For this review, use the dimensioned drawing (mm, ordinates from the lowest corner) and the shaded views. A direction names the side the tool comes from. Round coordinates to 2 decimals unless told otherwise and drop trailing zeros. Write each loop counter-clockwise with the first axis right and the second up, starting at its lowest first coordinate (ties: lowest second). Pieces come first, ordered by that corner, then holes. Notation, with made-up numbers: M 9,53 L 28,53 A22 cw 28,60 Z; hole C 10,9 d9. An arc over 180 degrees is marked long. One line per question, with ' | ' between items. Start each with the question number.
Item 1: For L1, parallel to X at y = 12.25, z = 15.5; L2, parallel to X at y = 0.55, z = 32, list the stretches that pass through material, from the lowest coordinate up.
Item 2: Machinability: for the marked faces 1 and 2, which of the approach directions +Z, -Z, +X, -X, +Y, -Y give a long, thin tool a straight path to every point of the face, cutting with its end or side? Answer none if there is none.
Item 3: Add section C-C, the plane y = 9.75. State the section outline as (x, z) points.
Item 4: Insertion check: pin 1 Ø5 at (y, z) = (16, 31.5) entering from -X; pin 2 Ø5.5 at (x, z) = (7, 57) entering from +Y. Each pin has a flat end and moves straight along its axis. Give the tip position at first contact, or say it passes through.
Item 5: Add section B-B, the plane x = 32. State the section outline as (y, z) points.
Item 6: Add section A-A, the plane z = 32. State the section outline as (x, y) points.
Item 7: Draft analysis for pull direction X (two halves, no side actions). For the marked faces 3, 4 and 5, state which applies: released by +X, released by -X, zero draft, split by the parting line, or undercut.
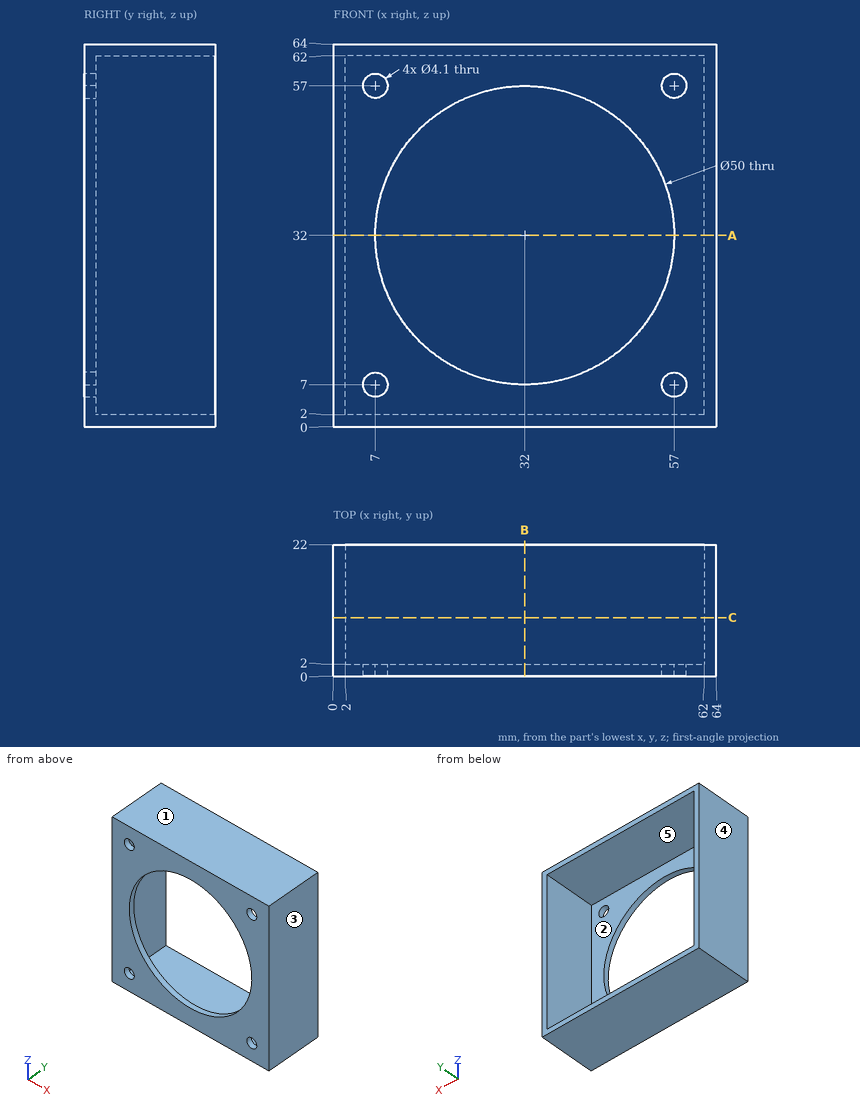
Computed values:
1) L1: x = 0 to 2, 62 to 64 | L2: x = 0 to 7, 57 to 64
2) face 1: +Z, +X, -X, +Y, -Y | face 2: +Y
3) outline: M 0,0 L 64,0 L 64,64 L 0,64 Z; hole M 2,2 L 62,2 L 62,62 L 2,62 Z
4) pin 1: stops at x = 0 | pin 2: stops at y = 2
5) outline: M 0,0 L 22,0 L 22,2 L 2,2 L 2,7 L 0,7 Z; M 0,57 L 2,57 L 2,62 L 22,62 L 22,64 L 0,64 Z
6) outline: M 0,0 L 7,0 L 7,2 L 2,2 L 2,22 L 0,22 Z; M 57,0 L 64,0 L 64,22 L 62,22 L 62,2 L 57,2 Z
7) face 3: released by +X | face 4: released by -X | face 5: undercut
